Part model, mm, in its own coordinate system. A direction names the side the tool comes from. Coordinates: 2 decimals unless noted, no trailing zeros. Write each loop counter-clockwise with the first axis right and the second up, starting at its lowest first coordinate (ties: lowest second). Pieces come first, ordered by that corner, then holes. Notation, with made-up numbers: (76.5, 2.5) - (107.5, 2.5) arc R14 cw to (107.5, 17.5) - close; hole circle Ø10 at (63.25, -13.5). An arc over 180 degrees is marked (long way). Use one line per item in the form item = value. Start each with the question number.
from build123d import *

# Parameters (mm, degrees)
SKETCH1_W           = 232
SKETCH1_H           = 380
BOSS_EXTRUDE1_DEPTH = 3
EXTRUDE_THIN1_DEPTH = 232


with BuildPart() as part:
    # Sketch1 → Boss-Extrude1 (new body)
    with BuildSketch(Plane(origin=(0, 0, 0), x_dir=(1, 0, 0), z_dir=(0, 1, 0))):
        Rectangle(SKETCH1_W, SKETCH1_H)
    extrude(amount=BOSS_EXTRUDE1_DEPTH)

    # Sketch5 → Extrude-Thin1 (add)
    with BuildSketch(Plane(origin=(116, 0, 0), x_dir=(0, 0, -1), z_dir=(1, 0, 0))):
        Polygon((190, 3), (242, -29), (240.427707723, -31.55497495), (188.427707723, 0.44502505), align=None)
    extrude(amount=-EXTRUDE_THIN1_DEPTH)


solid = part.part
Q1. Pin check, flat tips, straight feed: P1, Ø1, axis at x = -92, y = -18.5, coming from the +Z side; P2, Ø3, axis at x = -40, y = -24, coming from the -Z side; P3, Ø1, axis at x = 58.5, z = 5.5, coming from the -Y side. Stop position of each tip, or through.
Q2. Which spindle directions (+Z, -Z, +X, -X, +Y, -Y) get a long thin tool onto all of the face, cutting with end or side? Do faces 4 (the flat face through (-2, 0, -2)), 5 (the flat face through (2, -13, -216)). Say none if no direction does.
Q3. Slice it at A-A (x = 34.5). List the corners of the cut face in (y, z), plus the area to 3 significant figures.
Q4. Slice it at B-B (z = -83). List the corners of the cut face in (x, y), plus the area to 3 significant figures.
Q5. Drill centre lines: probe 1 along Y at (x, z) = (101, -113); probe 2 along Z at (x, y) = (-5, 0.5); probe 3 along Z at (x, y) = (78.5, -21). Where is each one in solid material? Low to high.
Q6. Slice it at C-C (y = -10). List the corners of the cut face in (x, z) (3 decimals), plus the area to 3 significant figures.
Q7. Mould opens along X. For faces 1 (the flat face through (1.62, -16, -215.15)), 2 (the flat face through (-116, 1, -27)), 3 (the flat face through (116, 1, -27)) say: released by +X, released by -X, zero draft, split by the parting line, or undercut.
Solution:
q1.P1 = -218.4
q1.P2 = -236.31
q1.P3 = 0
q2.face_4 = +Z, +X, -X, -Y
q2.face_5 = -Z, +X, -X, +Y
q3.outline = (-31.55, -240.43) - (-29, -242) - (3, -190) - (3, 190) - (0, 190) - (0, -189.15) - close
q3.area = 1,320 mm2
q4.outline = (-116, 0) - (116, 0) - (116, 3) - (-116, 3) - close
q4.area = 696 mm2
q5.probe_1 = 0 to 3
q5.probe_2 = -194.06 to 190
q5.probe_3 = -229 to -223.28
q6.outline = (-116, -211.125) - (116, -211.125) - (116, -205.401) - (-116, -205.401) - close
q6.area = 1,330 mm2
q7.face_1 = zero draft
q7.face_2 = released by -X
q7.face_3 = released by +X
